Geometry: see drawing. Coordinates: mm, zero at the bounding-box minimum. A direction names the side the tool comes from. Coordinates: 2 decimals unless noted, no trailing zeros. Write each loop counter-clockwise with the first axis right and the second up, starting at its lowest first coordinate (ties: lowest second). Pieces come first, ordered by that corner, then holes.
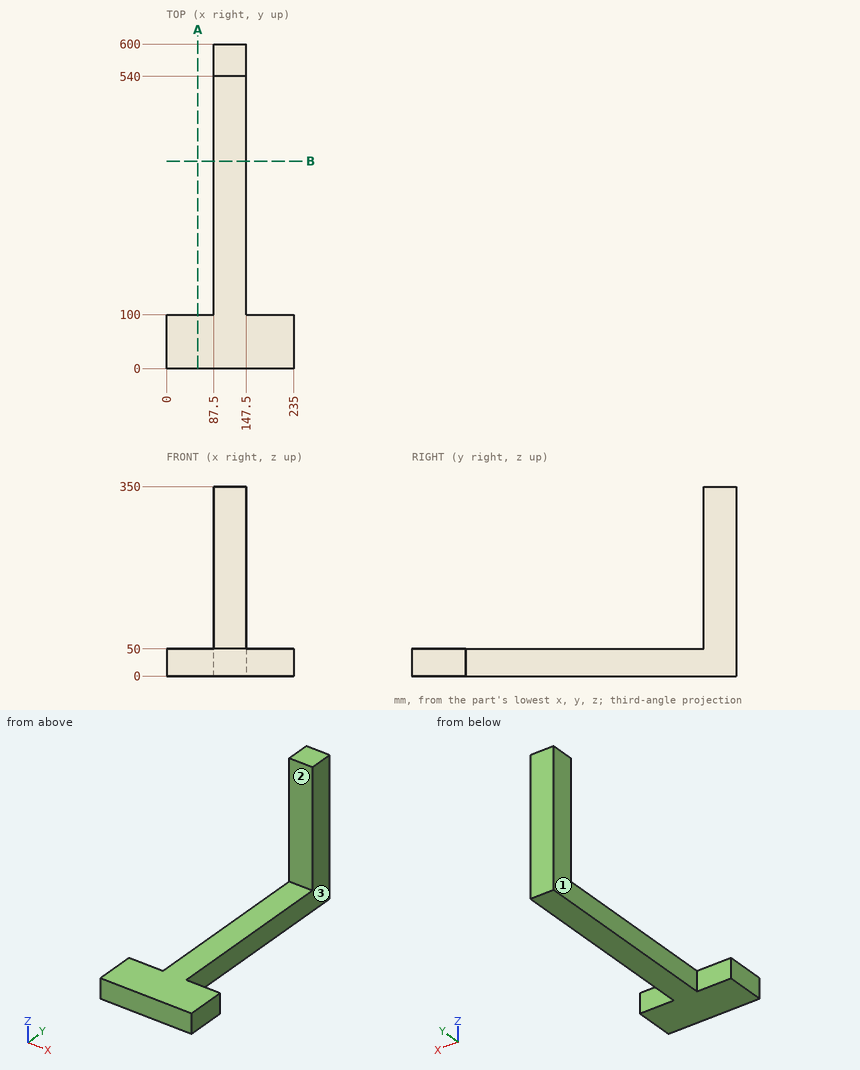
Item 1: Set-up query: the marked faces 1, 2 and 3. Return all of +Z, -Z, +X, -X, +Y, -Y with unobstructed straight access to the full face (end or side cutting, diameter ignored); none if empty.
Derived:
face 1: +Z, -Z, -X, +Y
face 2: +Z, +X, -X, -Y
face 3: +Z, -Z, +X, +Y
Item 2: Section A-A, the plane x = 58. Output: boundary loops of the cut face in (y, z), plus the area to 3 significant figures.
Derived:
outline: (0, 0) - (100, 0) - (100, 50) - (0, 50) - close
area: 5,000 mm2
Item 3: Material intervals for probe 1 along Y at (x, z) = (122, 185); probe 2 along Z at (x, y) = (142, 291), sorted ascending.
Derived:
probe 1: y = 540 to 600
probe 2: z = 0 to 50
Item 4: Section B-B, the plane y = 383.5. Output: boundary loops of the cut face in (x, z).
Derived:
outline: (87.5, 0) - (147.5, 0) - (147.5, 50) - (87.5, 50) - close
Item 5: Pin query (flat end, axial travel): pin 1 (1 mm diameter, centred on x = 148.5, z = 208.5, fed in from +Y); pin 2 (25 mm diameter, centred on x = 200.5, z = 25.5, fed in from +Y). Return the tip coordinate at first contact, or that it passes through.
Derived:
pin 1: passes through
pin 2: stops at y = 100
